```python
from build123d import *


with BuildPart() as part:
    # Model → Revolve1 (revolve)
    with BuildSketch(Plane.XY, mode=Mode.PRIVATE) as revolve1_sk:
        with BuildLine():
            Line((0, 47.573231), (117.474371, 47.573231))
            ThreePointArc((117.474371, 47.573231), (122.762513596, 46.877033869), (127.690278, 44.835887))
            Line((127.690278, 44.835887), (170.361247243, 20.199791421))
            ThreePointArc((170.361247243, 20.199791421), (176.44612601, 17.679352192), (182.976005243, 16.819677421))
            ThreePointArc((182.976005243, 16.819677421), (183.814650955, 16.874644956), (184.638947243, 17.038607421))
            Line((184.638947243, 17.038607421), (249.383859243, 34.386954421))
            Line((249.383859243, 34.386954421), (249.383859243, 69.85))
            Line((249.383859243, 69.85), (0, 69.85))
            Line((0, 69.85), (0, 47.573231))
        make_face()
    revolve(revolve1_sk.sketch.rotate(Axis((0, 0, 0), (1, 0, 0)), 90), axis=Axis((0, 0, 0), (1, 0, 0)))


solid = part.part
```
Check sheet for the modelled part. Datum: model origin and axes. Units: mm. A direction names the side the tool comes from. Coordinates: 2 decimals unless noted, no trailing zeros. Loops run counter-clockwise (first coordinate to the right, second up) from the corner with the lowest first, then second, coordinate; pieces in that order, holes last.
1) Sectioned sample at C-C (x = 23). Record the boundary of the cut face in (y, z).
2) Material ranges on probe 1 along Y at (x, z) = (84, 2); probe 2 along Y at (x, z) = (40.5, 0); probe 3 along Z at (x, y) = (97, 26.5), recorded low to high.
3) Gauge pin test, flat ends, axial feed: pin 1 (5 mm diameter, centred on x = 215, z = 2.5, fed in from -Y); pin 2 (3 mm diameter, centred on x = 37.5, y = -55, fed in from -Z); pin 3 (8 mm diameter, centred on x = 175, z = -21.5, fed in from -Y). Record the tip position at first contact, or that the pin passes through.
4) Sectioned sample at D-D (y = 60.5). Record the boundary of the cut face in (x, z), and give its area (3 significant figures).
5) Release check for a two-part mould opening along Z. For faces 3 (the face through (249.384, -32, -15)), 4 (the face through (163.548, 14.685, -19.151)), 5 (the face through (122.9, 68.2, -15.1)) record: released by +Z, released by -Z, zero draft, split by the parting line, or undercut.
6) Sectioned sample at A-A (z = 0). Record the boundary of the cut face in (x, y), and give its area (3 significant figures).
7) Access from +Z, -Z, +X, -X, +Y, -Y to the whole of each face (thin tool, end or side, straight path). Record for faces 1 (the face through (210.271, -7.181, 22.803)), 2 (the face through (59.56, -47.17, -6.19)).
Check sheet entries:
1. outline: circle Ø139.7 at (0, 0); hole circle Ø95.15 at (0, 0)
2. probe 1: y = -69.82 to -47.53, 47.53 to 69.82
2. probe 2: y = -69.85 to -47.57, 47.57 to 69.85
2. probe 3: z = -64.63 to -39.51, 39.51 to 64.63
3. pin 1: stops at y = -69.85
3. pin 2: stops at z = -44.91
3. pin 3: stops at y = -67.62
4. outline: (0, -34.91) - (249.38, -34.91) - (249.38, 34.91) - (0, 34.91) - close
4. area: 17,400 mm2
5. face 3: zero draft
5. face 4: undercut
5. face 5: split by the parting line
6. outline: (0, -69.85) - (249.38, -69.85) - (249.38, -34.39) - (184.64, -17.04) arc R6.43 ccw to (182.98, -16.82) arc R25.23 ccw to (170.36, -20.2) - (127.69, -44.84) arc R20.43 cw to (117.47, -47.57) - (0, -47.57) - close; (0, 47.57) - (117.47, 47.57) arc R20.43 cw to (127.69, 44.84) - (170.36, 20.2) arc R25.23 ccw to (182.98, 16.82) arc R6.43 ccw to (184.64, 17.04) - (249.38, 34.39) - (249.38, 69.85) - (0, 69.85) - close
6. area: 16,100 mm2
7. face 1: +X
7. face 2: -X
